from build123d import *

# Parameters (mm, degrees)
SKETCH_1_R          = 1.05
SKETCH_1_R_2        = 1.55
EXTRUDE_1_DEPTH     = 6
SKETCH_2_R          = 1.55
CUT_EXTRUDE_1_DEPTH = 3
CUT_EXTRUDE_2_DEPTH = 75.242844773
CUT_EXTRUDE_3_DEPTH = 4
SKETCH_6_R          = 1.9
CUT_EXTRUDE_4_DEPTH = 3
SKETCH_7_W          = 6
SKETCH_7_H          = 0.01
EXTRUDE_2_DEPTH     = 4


with BuildPart() as part:
    # ｽｹｯﾁ1 → ﾎﾞｽ - 押し出し1 (new body)
    with BuildSketch(Plane.XY):
        with BuildLine():
            Line((-11, 4.6), (-11, 24))
            Line((-11, 24), (-17.5, 24))
            Line((-17.5, 24), (-70, 2))
            Line((-70, 2), (-70, -4))
            Line((-70, -4), (-17.5, -4))
            Line((-17.5, -4), (17.5, -4))
            Line((17.5, -4), (70, -4))
            Line((70, -4), (70, 2))
            Line((70, 2), (17.5, 24))
            Line((17.5, 24), (11, 24))
            Line((11, 24), (11, 4.6))
            ThreePointArc((11, 4.6), (10.38492424, 3.11507576), (8.9, 2.5))
            Line((8.9, 2.5), (-8.9, 2.5))
            ThreePointArc((-8.9, 2.5), (-10.38492424, 3.11507576), (-11, 4.6))
        make_face()
        with Locations((-13.5, 5.5)):
            Circle(SKETCH_1_R, mode=Mode.SUBTRACT)
        with Locations((-8, 0)):
            Circle(SKETCH_1_R, mode=Mode.SUBTRACT)
        with Locations((8, 0)):
            Circle(SKETCH_1_R, mode=Mode.SUBTRACT)
        with Locations((-13.5, 13.5)):
            Circle(SKETCH_1_R, mode=Mode.SUBTRACT)
        with Locations((-13.5, 21.5)):
            Circle(SKETCH_1_R, mode=Mode.SUBTRACT)
        with Locations((13.5, 21.5)):
            Circle(SKETCH_1_R, mode=Mode.SUBTRACT)
        with Locations((13.5, 13.5)):
            Circle(SKETCH_1_R, mode=Mode.SUBTRACT)
        with Locations((13.5, 5.5)):
            Circle(SKETCH_1_R, mode=Mode.SUBTRACT)
        with Locations((-65, -1)):
            Circle(SKETCH_1_R_2, mode=Mode.SUBTRACT)
        with Locations(Location((65, -1, 0), (0, 0, 180))):
            Circle(SKETCH_1_R_2, mode=Mode.SUBTRACT)
        with BuildLine():
            Line((-17.5, 4.1), (-17.5, 16.506066998))
            ThreePointArc((-17.5, 16.506066998), (-18.436901101, 18.254552329), (-20.411619954, 18.442887344))
            Line((-20.411619954, 18.442887344), (-50.017007109, 6.036820345))
            ThreePointArc((-50.017007109, 6.036820345), (-51.264188108, 3.686069284), (-49.205387155, 2))
            Line((-49.205387155, 2), (-19.6, 2))
            ThreePointArc((-19.6, 2), (-18.11507576, 2.61507576), (-17.5, 4.1))
        make_face(mode=Mode.SUBTRACT)
        with BuildLine():
            Line((20.411619954, 18.442887344), (50.017007109, 6.036820345))
            ThreePointArc((50.017007109, 6.036820345), (51.264188108, 3.686069284), (49.205387155, 2))
            Line((49.205387155, 2), (19.6, 2))
            ThreePointArc((19.6, 2), (18.11507576, 2.61507576), (17.5, 4.1))
            Line((17.5, 4.1), (17.5, 16.506066998))
            ThreePointArc((17.5, 16.506066998), (18.436901101, 18.254552329), (20.411619954, 18.442887344))
        make_face(mode=Mode.SUBTRACT)
    extrude(amount=EXTRUDE_1_DEPTH)

    # ｽｹｯﾁ2 → ｶｯﾄ - 押し出し1 (cut)
    with BuildSketch(Plane.XY.offset(6)):
        with Locations((-48, -1)):
            Circle(SKETCH_2_R)
        with Locations(Location((48, -1, 0), (0, 0, 180))):
            Circle(SKETCH_2_R)
        with Locations((-58, -1)):
            Circle(SKETCH_2_R)
        with Locations(Location((58, -1, 0), (0, 0, 180))):
            Circle(SKETCH_2_R)
    extrude(amount=-CUT_EXTRUDE_1_DEPTH, mode=Mode.SUBTRACT)

    # ｽｹｯﾁ3 → ｶｯﾄ - 押し出し2 (cut, through all)
    with BuildSketch(Plane(origin=(0, 0, 0), x_dir=(-1, 0, 0), z_dir=(0, 0, -1))):
        with BuildLine():
            Line((-56.45, -0.75), (-56.45, -1.25))
            ThreePointArc((-56.45, -1.25), (-58, -2.8), (-59.55, -1.25))
            Line((-59.55, -1.25), (-59.55, -0.75))
            ThreePointArc((-59.55, -0.75), (-58, 0.8), (-56.45, -0.75))
        make_face()
        with BuildLine():
            Line((-46.45, -0.75), (-46.45, -1.25))
            ThreePointArc((-46.45, -1.25), (-48, -2.8), (-49.55, -1.25))
            Line((-49.55, -1.25), (-49.55, -0.75))
            ThreePointArc((-49.55, -0.75), (-48, 0.8), (-46.45, -0.75))
        make_face()
        with BuildLine():
            Line((56.45, -0.75), (56.45, -1.25))
            ThreePointArc((56.45, -1.25), (58, -2.8), (59.55, -1.25))
            Line((59.55, -1.25), (59.55, -0.75))
            ThreePointArc((59.55, -0.75), (58, 0.8), (56.45, -0.75))
        make_face()
        with BuildLine():
            Line((46.45, -0.75), (46.45, -1.25))
            ThreePointArc((46.45, -1.25), (48, -2.8), (49.55, -1.25))
            Line((49.55, -1.25), (49.55, -0.75))
            ThreePointArc((49.55, -0.75), (48, 0.8), (46.45, -0.75))
        make_face()
    extrude(amount=-CUT_EXTRUDE_2_DEPTH, mode=Mode.SUBTRACT)

    # ｽｹｯﾁ4 → ｶｯﾄ - 押し出し3 (cut)
    with BuildSketch(Plane(origin=(0, 0, 0), x_dir=(-1, 0, 0), z_dir=(0, 0, -1))):
        with BuildLine():
            Line((-68, -1), (-68, -4))
            Line((-68, -4), (-62, -4))
            Line((-62, -4), (-62, -1))
            ThreePointArc((-62, -1), (-65, 2), (-68, -1))
        make_face()
        with BuildLine():
            Line((62, -4), (62, -1))
            ThreePointArc((62, -1), (65, 2), (68, -1))
            Line((68, -1), (68, -4))
            Line((68, -4), (62, -4))
        make_face()
    extrude(amount=-CUT_EXTRUDE_3_DEPTH, mode=Mode.SUBTRACT)

    # ｽｹｯﾁ6 → ｶｯﾄ - 押し出し4 (cut)
    with BuildSketch(Plane(origin=(0, 0, 0), x_dir=(-1, 0, 0), z_dir=(0, 0, -1))):
        with Locations((-13.5, 21.5)):
            Circle(SKETCH_6_R)
        with Locations((-13.5, 13.5)):
            Circle(SKETCH_6_R)
        with Locations((-13.5, 5.5)):
            Circle(SKETCH_6_R)
        with Locations((-8, 0)):
            Circle(SKETCH_6_R)
        with Locations(Location((8, 0, 0), (0, 0, 180))):
            Circle(SKETCH_6_R)
        with Locations(Location((13.5, 5.5, 0), (0, 0, 180))):
            Circle(SKETCH_6_R)
        with Locations(Location((13.5, 13.5, 0), (0, 0, 180))):
            Circle(SKETCH_6_R)
        with Locations(Location((13.5, 21.5, 0), (0, 0, 180))):
            Circle(SKETCH_6_R)
    extrude(amount=-CUT_EXTRUDE_4_DEPTH, mode=Mode.SUBTRACT)

    # ｽｹｯﾁ7 → ﾎﾞｽ - 押し出し2 (add)
    with BuildSketch(Plane(origin=(0, 0, 4), x_dir=(-1, 0, 0), z_dir=(0, 0, -1))):
        with Locations((65, -3.995)):
            Rectangle(SKETCH_7_W, SKETCH_7_H)
        with Locations((-65, -3.995)):
            Rectangle(SKETCH_7_W, SKETCH_7_H)
    extrude(amount=EXTRUDE_2_DEPTH)


solid = part.part
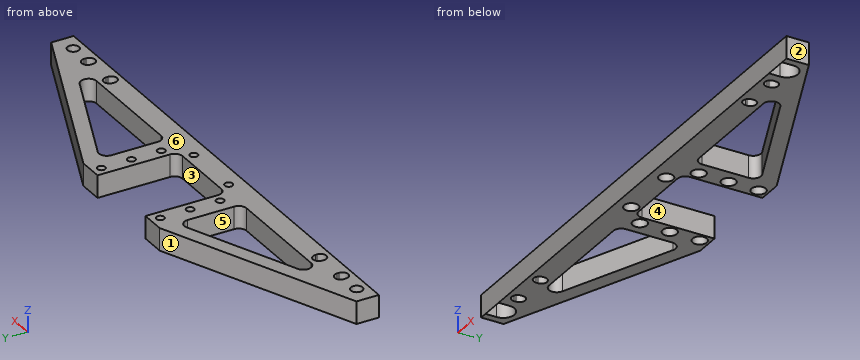
Can you work these out from the model? Positions are in its coordinate system, mm. Face numbers are marked on the shaded views. A direction names the side the tool comes from. Round coordinates to 2 decimals unless told otherwise and drop trailing zeros. Loops run counter-clockwise (first coordinate to the right, second up) from the corner with the lowest first, then second, coordinate; pieces in that order, holes last. Notation, with made-up numbers: (-11, 45) - (23, 45) arc R8 cw to (23, 51) - close; hole circle Ø4 at (43, 19). An arc over 180 degrees is marked (long way). Write item = value, one per line. Start each with the question number.
(1) If we section it at A-A (x = -48): Please give me the cut outline in (y, z).
(2) If we mould it in two halves opening along X, with no side actions, what happens to the marked faces 1, 2 and 3? For each: released by +X, released by -X, zero draft, split by the parting line, or undercut.
(3) If we section it at C-C (z = 5.05): Give the number of separate pieces and of enclosed holes in the cut face, and give its area (3 significant figures).
(4) For P1, Ø1.9, axis at x = -13.5, y = 6, coming from the -Z side; P2, Ø1.8, axis at y = 8.5, z = 3, coming from the -X side; P3, Ø1, axis at y = 5, z = 4.5, coming from the +X side, each with a flat end and sliding along its axis, tell me the tip position at first contact or that it passes through.
(5) If we section it at D-D (x = 58): Please give me the cut outline in (y, z).
(6) If I drill on probe 1 along Y at (x, z) = (-13.5, 1.5); probe 2 along Y at (x, z) = (-13.5, 4.45); probe 3 along X at (y, z) = (8.75, 4.8), over which ranges is the centre line in solid material (lowest first)? Write a range as [from, to].
(7) For the marked faces 4, 5 and 6, which set-ups out of +Z, -Z, +X, -X, +Y, -Y let a thin tool reach every point of the face, with its end or its side?
Ans:
q1.outline = (-4, 0) - (-2.8, 0) - (-2.8, 6) - (-4, 6) - close; (0.8, 0) - (2, 0) - (2, 6) - (0.8, 6) - close; (6.88, 0) - (11.22, 0) - (11.22, 6) - (6.88, 6) - close
q2.face_1 = released by -X
q2.face_2 = released by +X
q2.face_3 = undercut
q3.separate_pieces = 1
q3.enclosed_holes = 16
q3.area = 1,510 mm²
q4.P1 = 3
q4.P2 = -56.64
q4.P3 = 64.03
q5.outline = (-4, 0) - (-2.8, 0) - (-2.8, 6) - (-4, 6) - close; (0.8, 0) - (7.03, 0) - (7.03, 6) - (0.8, 6) - close
q6.probe_1 = [-4, 3.6], [7.4, 11.6], [15.4, 19.6], [23.4, 24]
q6.probe_2 = [-4, 4.45], [6.55, 12.45], [14.55, 20.45], [22.55, 24]
q6.probe_3 = [-53.89, -43.54], [-17.5, -11], [11, 17.5], [43.54, 53.89]
q7.face_4 = +Z, -Z, +Y
q7.face_5 = +Z, -Z
q7.face_6 = +Z, +X, -X, +Y, -Y
